Build history of the part. All positions in model axes, mm. Face numbers are marked on the shaded views. A direction names the side the tool comes from. Round coordinates to 2 decimals unless told otherwise and drop trailing zeros. Loops run counter-clockwise (first coordinate to the right, second up) from the corner with the lowest first, then second, coordinate; pieces in that order, holes last. Notation, with made-up numbers: (-38, 82) -> (-28, 82) arc R38 ccw to (-28, 120) -> close; hole circle Ø4 at (5, -8). An arc over 180 degrees is marked (long way). Put each result on its own line as item: value. Start each with the question number.
Item 1: Cut at D-D, the plane z = 8. List the corners of the cut face in (x, y), plus the area to 3 significant figures.
Item 2: Tool access for the marked faces 1 and 2: list every direction of +Z, -Z, +X, -X, +Y, -Y with a clear straight run to the whole face (end or side of a thin tool).
Item 3: Cut at A-A, the plane z = 0. List the corners of the cut face in (x, y).
Item 4: Drill centre lines: probe 1 along Y at (x, z) = (7.5, 3); probe 2 along X at (y, z) = (-70, 0.75); probe 3 along Z at (x, y) = (-1, -64). Where is each one in solid material? Low to high. Write a range as [from, to].
Item 5: Flat gauge pins, fed straight in: pin 1 Ø4 at (x, y) = (0.5, -31) entering from +Z; pin 2 Ø2 at (y, z) = (-48, 4.5) entering from +X; pin 3 Ø3 at (y, z) = (-57, -2.5) entering from +X; pin 4 Ø1.5 at (x, y) = (7.5, -1) entering from +Z. Where does each tip first touch, or does it go through?
Item 6: Cut at C-C, the plane y = -54.5. List the corners of the cut face in (x, z), plus the area to 3 significant figures.
Item 7: Cut at B-B, the plane x = 0. List the corners of the cut face in (y, z), plus the area to 3 significant figures.
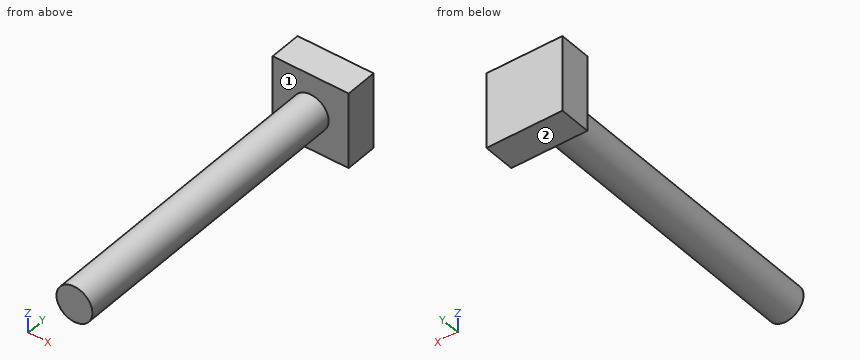
```python
from build123d import *

# Parameters (mm, degrees)
SKETCH3_W           = 19
SKETCH3_H           = 19
BOSS_EXTRUDE1_DEPTH = 8
SKETCH4_R           = 4.5
BOSS_EXTRUDE2_DEPTH = 76


with BuildPart() as part:
    # Sketch3 → Boss-Extrude1 (new body)
    with BuildSketch(Plane(origin=(0, 0, 0), x_dir=(1, 0, 0), z_dir=(0, 1, 0))):
        Rectangle(SKETCH3_W, SKETCH3_H)
    extrude(amount=BOSS_EXTRUDE1_DEPTH)

    # Sketch4 → Boss-Extrude2 (add)
    with BuildSketch(Plane(origin=(0, 0, 0), x_dir=(1, 0, 0), z_dir=(0, 1, 0))):
        with Locations(Location((0, 0, 0), (0, 0, 270))):  # turned: the seam where the file's is
            Circle(SKETCH4_R)
    extrude(amount=-BOSS_EXTRUDE2_DEPTH)


solid = part.part
```
Reply:
1. outline: (-9.5, 0) -> (9.5, 0) -> (9.5, 8) -> (-9.5, 8) -> close
1. area: 152 mm^2
2. face 1: -Y
2. face 2: -Z, +X, -X, +Y, -Y
3. outline: (-9.5, 0) -> (-4.5, 0) -> (-4.5, -76) -> (4.5, -76) -> (4.5, 0) -> (9.5, 0) -> (9.5, 8) -> (-9.5, 8) -> close
4. probe 1: y = [0, 8]
4. probe 2: x = [-4.44, 4.44]
4. probe 3: z = [-4.39, 4.39]
5. pin 1: stops at z = 4.5
5. pin 2: stops at x = 2.83
5. pin 3: stops at x = 4.39
5. pin 4: passes through
6. outline: circle Ø9 at (0, 0)
6. area: 63.6 mm^2
7. outline: (-76, -4.5) -> (0, -4.5) -> (0, -9.5) -> (8, -9.5) -> (8, 9.5) -> (0, 9.5) -> (0, 4.5) -> (-76, 4.5) -> close
7. area: 836 mm^2
